Here's how the part is built. I have some questions about the finished solid (model axes, mm). Face numbers are marked on the shaded views. A direction names the side the tool comes from. Give positions to 0.01 mm unless a question says otherwise; leave off trailing zeros. Loops run counter-clockwise (first coordinate to the right, second up) from the corner with the lowest first, then second, coordinate; pieces in that order, holes last.
Q1. I need wall thicknesses on line 1 (X direction, y = 10, z = 11.75); line 2 (Y direction, x = 9, z = 9.5); line 3 (Y direction, x = 6.75, z = 16.5). Which ranges of each line are inside material? Lowest first, please.
Q2. For the marked faces 1, 2 and 3, which set-ups out of +Z, -Z, +X, -X, +Y, -Y let a thin tool reach every point of the face, with its end or its side?
Q3. If we section it at B-B (y = 16.5): Please give me the cut outline in (x, z).
Q4. If we section it at A-A (x = 14.25): Please give me the cut outline in (y, z), plus the area to 3 significant figures.
Q5. Will these pins go through, and if not, where does the flat tip stop? P1, Ø5, axis at x = -3.5, z = 5, coming from the -Y side; P2, Ø8, axis at x = 5, z = 4.5, coming from the +Y side; P3, Ø8, axis at y = 20.5, z = 7, coming from the -X side.
Q6. If we section it at C-C (z = 3): Please give me the cut outline in (x, y), plus the area to 4 significant figures.
Q7. If we section it at D-D (x = 4): Please give me the cut outline in (y, z), plus the area to 3 significant figures.
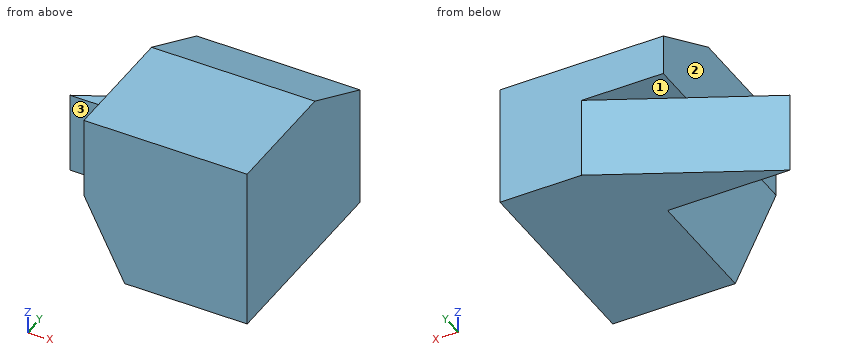
from build123d import *

# Parameters (mm, degrees)
SKETCH1_W           = 20
SKETCH1_H           = 25
BOSS_EXTRUDE1_DEPTH = 20
CUT_EXTRUDE1_DEPTH  = 20
SKETCH4_W           = 10
SKETCH4_H           = 10
BOSS_EXTRUDE2_DEPTH = 10
CUT_EXTRUDE2_DEPTH  = 50
CUT_EXTRUDE3_DEPTH  = 15


with BuildPart() as part:
    # Sketch1 → Boss-Extrude1 (new body)
    with BuildSketch(Plane.XY):
        with Locations((10, 12.5)):
            Rectangle(SKETCH1_W, SKETCH1_H)
    extrude(amount=BOSS_EXTRUDE1_DEPTH)

    # Sketch3 → Cut-Extrude1 (cut)
    with BuildSketch(Plane.ZY):
        Polygon((15, 25), (20, 15), (20, 25), align=None)
    extrude(amount=-CUT_EXTRUDE1_DEPTH, mode=Mode.SUBTRACT)

    # Sketch4 → Boss-Extrude2 (add)
    with BuildSketch(Plane.ZY):
        with Locations((5, 20)):
            Rectangle(SKETCH4_W, SKETCH4_H)
    extrude(amount=BOSS_EXTRUDE2_DEPTH)

    # Sketch5 → Cut-Extrude2 (cut)
    with BuildSketch(Plane.XY.offset(10)):
        Polygon((-10, 15), (10, 25), (-10, 25), align=None)
    extrude(amount=-CUT_EXTRUDE2_DEPTH, mode=Mode.SUBTRACT)

    # Sketch6 → Cut-Extrude3 (cut)
    with BuildSketch(Plane.XZ):
        Polygon((0, 10), (5, 0), (0, 0), align=None)
    extrude(amount=-CUT_EXTRUDE3_DEPTH, mode=Mode.SUBTRACT)


solid = part.part
Check sheet entries:
1. line 1: x = 0 to 20
1. line 2: y = 0 to 24.5
1. line 3: y = 0 to 22
2. face 1: -Z, -X, +Y
2. face 2: +Z, -X, +Y, -Y
2. face 3: -Z, -X, -Y
3. outline: (-7, 0) - (20, 0) - (20, 19.25) - (0, 19.25) - (0, 10) - (-7, 10) - close
4. outline: (0, 0) - (25, 0) - (25, 15) - (15, 20) - (0, 20) - close
4. area: 475 mm2
5. P1: stops at y = 15
5. P2: stops at y = 24.5
5. P3: stops at x = -7
6. outline: (-10, 15) - (3.5, 15) - (3.5, 0) - (20, 0) - (20, 25) - (10, 25) - close
6. area: 447.5 mm2
7. outline: (0, 2) - (15, 2) - (15, 0) - (22, 0) - (22, 10) - (25, 10) - (25, 15) - (15, 20) - (0, 20) - close
7. area: 415 mm2
